from build123d import *

# Parameters (mm, degrees)
PAD_DEPTH    = 30
SKETCH001_R  = 7.5
POCKET_DEPTH = 5
FILLET_R     = 5


with BuildPart() as part:
    # Sketch → Pad (new body)
    with BuildSketch(Plane.XY):
        Polygon((0, 0), (0, 43), (47.1, 43), (47.1, 40), (10.1, 40), (10.1, 0), (7.1, 0), (7.1, 38), (3, 38), (3, 0), align=None)
    extrude(amount=PAD_DEPTH)

    # Sketch001 (on Face2 of Pad) → Pocket (cut)
    with BuildSketch(Plane(origin=(0, 43, 0), x_dir=(-1, 0, 0), z_dir=(0, 1, 0))):
        with Locations((-32.1, 15)):
            Circle(SKETCH001_R)
    extrude(amount=-POCKET_DEPTH, mode=Mode.SUBTRACT)

    # Fillet
    fillet_edges = [part.edges().sort_by_distance(p)[0] for p in [
        (47.1, 41.5, 0),
        (47.1, 41.5, 30),
    ]]
    fillet(fillet_edges, radius=FILLET_R)


solid = part.part
Geometry check sheet. Reference: the model listing, model coordinates, mm. A direction names the side the tool comes from. Round coordinates to 2 decimals unless told otherwise and drop trailing zeros. Write each loop counter-clockwise with the first axis right and the second up, starting at its lowest first coordinate (ties: lowest second). Pieces come first, ordered by that corner, then holes.
Item 1: Section check C-C (z = 11.5). Record the boundary of the cut face in (x, y).
Determined:
outline: (0, 0) - (3, 0) - (3, 38) - (7.1, 38) - (7.1, 0) - (10.1, 0) - (10.1, 40) - (25.47, 40) - (25.47, 43) - (0, 43) - close; (38.73, 40) - (47.1, 40) - (47.1, 43) - (38.73, 43) - close
Item 2: Material ranges on line 1 along X through (y, z) = (34, 26.25); line 2 along Z through (x, y) = (32.1, 42.05); line 3 along Y through (x, z) = (44, 27.25), recorded low to high.
Determined:
line 1: x = 0 to 3, 7.1 to 10.1
line 2: z = 0 to 7.5, 22.5 to 30
line 3: y = 40 to 43
Item 3: Section check A-A (x = 32.1). Record the boundary of the cut face in (y, z).
Determined:
outline: (40, 0) - (43, 0) - (43, 7.5) - (40, 7.5) - close; (40, 22.5) - (43, 22.5) - (43, 30) - (40, 30) - close
Item 4: Section check D-D (z = 15). Record the boundary of the cut face in (x, y).
Determined:
outline: (0, 0) - (3, 0) - (3, 38) - (7.1, 38) - (7.1, 0) - (10.1, 0) - (10.1, 40) - (24.6, 40) - (24.6, 43) - (0, 43) - close; (39.6, 40) - (47.1, 40) - (47.1, 43) - (39.6, 43) - close
Item 5: Mould release check, pull along X, two halves, no side actions. Record for faces 1 (the face through (5, 38, 15)), 2 (the face through (45.6, 41.48, 1.43)), 3 (the face through (9, 28, 30)): +X half, -X half, draft (parallel to the pull), parting line (faces both ways), or undercut.
Determined:
face 1: undercut
face 2: +X half
face 3: draft
Item 6: Access from +Z, -Z, +X, -X, +Y, -Y to the whole of each face (thin tool, end or side, straight path). Record for faces 4 (the face through (10.1, 20, 15)), 5 (the face through (47.1, 42, 15)), 6 (the face through (3, 19, 15)).
Determined:
face 4: +Z, -Z, +X, -Y
face 5: +Z, -Z, +X, +Y, -Y
face 6: +Z, -Z, -Y
Item 7: Section check B-B (y = 37). Record the boundary of the cut face in (x, z), plus the area to 3 significant figures.
Determined:
outline: (0, 0) - (3, 0) - (3, 30) - (0, 30) - close; (7.1, 0) - (10.1, 0) - (10.1, 30) - (7.1, 30) - close
area: 180 mm2
Item 8: Go/stop test with flat-tipped pins: pin 1 Ø10 at (x, y) = (19, 15) entering from -Z; pin 2 Ø9 at (x, z) = (25, 12.5) entering from -Y; pin 3 Ø8 at (y, z) = (18.5, 9) entering from +X; pin 4 Ø3.5 at (x, z) = (5, 15) entering from -Y. Record where each tip stops, or that it passes through.
Determined:
pin 1: passes through
pin 2: stops at y = 40
pin 3: stops at x = 10.1
pin 4: stops at y = 38
